Check sheet for the modelled part. Datum: model origin and axes. Units: mm. Face numbers are marked on the shaded views. A direction names the side the tool comes from. Round coordinates to 2 decimals unless told otherwise and drop trailing zeros. Order: outer loops, then holes, each group sorted by start corner. A loop starts at its lowest first (then second) coordinate and runs counter-clockwise, first axis right, second up.
(1) Sectioned sample at C-C, the plane y = -43. Enter the section's corners in (x, z), and give its area (3 significant figures).
(2) Sectioned sample at A-A, the plane x = -88. Enter the section's corners in (y, z), and give its area (3 significant figures).
(3) Sectioned sample at B-B, the plane y = 44.5. Enter the section's corners in (x, z).
(4) Mould release check, pull along X, two halves, no side actions. Record for the marked faces 1, 2, 3 and 4: released by +X, released by -X, zero draft, split by the parting line, or undercut.
(5) Thickness scan on probe 1 along X at (y, z) = (8.5, 15.75); probe 2 along X at (y, z) = (9.5, 5.25); probe 3 along Y at (x, z) = (9, 4). Record the ranges inside material, lowest first.
(6) Tool access check on the marked faces 5 and 6. Record the directions out of +Z, -Z, +X, -X, +Y, -Y that give a thin tool (end or side, any length) a straight path to the whole face; none if there is none.
(7) Depth check by flat-ended pin: pin 1 (6 mm diameter, centred on y = 27, z = 8.5, fed in from +X); pin 2 (10 mm diameter, centred on x = -4, z = 8, fed in from -Y); pin 3 (12.5 mm diameter, centred on y = -2.5, z = 11, fed in from +X). Enter the tip coordinate at first touch or a pass-through.
```python
from build123d import *

# Parameters (mm, degrees)
F0_R     = 13.97
F1_DEPTH = 25.4
F2_R     = 5.08
F3_R     = 3.175
F4_DEPTH = 5.001
F5_R     = 9.573934


with BuildPart() as f1:
    # F0 (on Top) → F1 (new body)
    with BuildSketch(Plane.XY):
        with BuildLine():
            Line((-127, 52.264305), (-132, 52.264305))
            Line((-132, 52.264305), (-132, -60.940004))
            Line((-132, -60.940004), (-127, -60.940004))
            Line((-127, -60.940004), (-127, -41.890004))
            Line((-127, -41.890004), (-1.012586, 3.965665))
            ThreePointArc((-1.012586, 3.965665), (32.5077, 24.635271), (-6.449811, 30.393267))
            Line((-6.449811, 30.393267), (-127, 33.214305))
            Line((-127, 33.214305), (-127, 52.264305))
        make_face()
        with BuildLine():
            Line((-127, -23.931264), (-127, 14.562711))
            ThreePointArc((-127, 14.562711), (-125.140128, 19.052839), (-120.65, 20.912711))
            Line((-120.65, 20.912711), (-35.507844, 20.912711))
            ThreePointArc((-35.507844, 20.912711), (-31.865634, 19.764326), (-29.540796, 16.734538))
            Line((-29.540796, 16.734538), (-27.128811, 10.107665))
            ThreePointArc((-27.128811, 10.107665), (-27.340805, 5.252211), (-30.924032, 1.968789))
            Line((-30.924032, 1.968789), (-118.478172, -29.898312))
            ThreePointArc((-118.478172, -29.898312), (-124.29221, -29.132879), (-127, -23.931264))
        make_face(mode=Mode.SUBTRACT)
        with Locations((11.979175, 20.411724)):
            Circle(F0_R, mode=Mode.SUBTRACT)
    extrude(amount=F1_DEPTH)

    # F2
    f2_edges = [f1.edges().sort_by_distance(p)[0] for p in [
        (-129.5, 52.264305, 25.4),
        (-129.5, 52.264305, 0),
        (-129.5, -60.940004, 0),
        (-129.5, -60.940004, 25.4),
    ]]
    fillet(f2_edges, radius=F2_R)

    # F3 (on face) → F4 (cut, through all)
    with BuildSketch(Plane.YZ.offset(-127)):
        with Locations((45.914305, 12.7)):
            Circle(F3_R)
        with Locations((-54.590004, 12.163277)):
            Circle(F3_R)
    extrude(amount=-F4_DEPTH, mode=Mode.SUBTRACT)

    # F5
    f5_edges = [f1.edges().sort_by_distance(p)[0] for p in [
        (-127, -41.890004, 12.7),
        (-127, 33.214305, 12.7),
    ]]
    fillet(f5_edges, radius=F5_R)


solid = f1.part
```
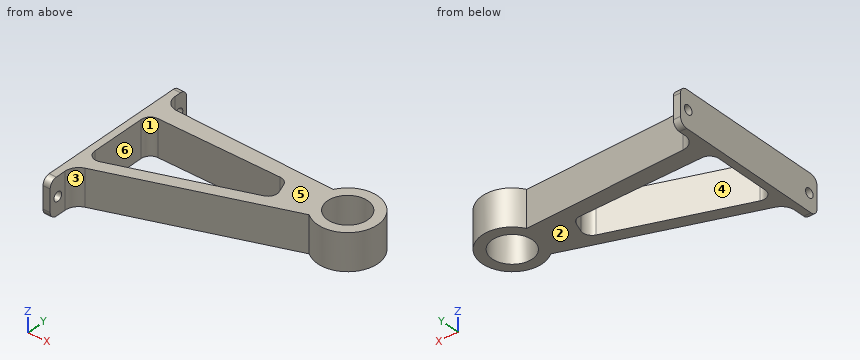
Derived:
1. outline: (-132, 0) - (-125.2, 0) - (-125.2, 25.4) - (-132, 25.4) - close
1. area: 173 mm2
2. outline: (-27.7, 0) - (-18.81, 0) - (-18.81, 25.4) - (-27.7, 25.4) - close; (20.91, 0) - (32.3, 0) - (32.3, 25.4) - (20.91, 25.4) - close
2. area: 515 mm2
3. outline: (-132, 0) - (-127, 0) - (-127, 9.86) - (-132, 9.86) - close; (-132, 15.54) - (-127, 15.54) - (-127, 25.4) - (-132, 25.4) - close
4. face 1: undercut
4. face 2: zero draft
4. face 3: released by +X
4. face 4: undercut
5. probe 1: x = -132 to -127, -26.77 to 4.68, 19.28 to 29.22
5. probe 2: x = -132 to -127, -26.94 to 3.26, 20.7 to 29.87
5. probe 3: y = -0.33 to 6.76, 34.06 to 41.16
6. face 5: +Z, +X, -X, +Y, -Y
6. face 6: +Z, -Z
7. pin 1: stops at x = 32.63
7. pin 2: stops at y = 1.06
7. pin 3: stops at x = 24.69
